Here's the drawing with two shaded views (mm, measured from the low corner). I have some questions. A direction names the side the tool comes from. Give positions to 0.01 mm unless a question says otherwise; leave off trailing zeros. Write each loop counter-clockwise with the first axis right and the second up, starting at its lowest first coordinate (ties: lowest second). Pieces come first, ordered by that corner, then holes.
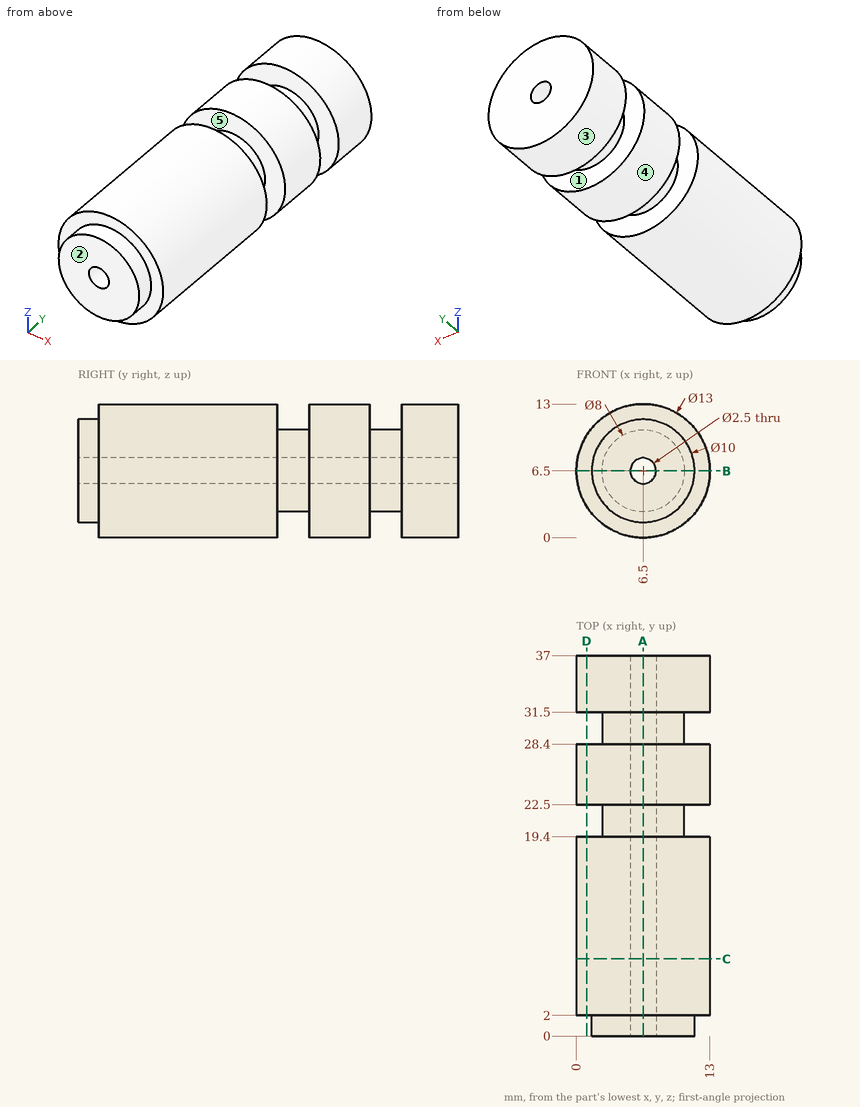
1) For pin 1 Ø1 at (y, z) = (30.5, 10) entering from -X; pin 2 Ø1.5 at (x, y) = (8.5, 26.5) entering from -Z; pin 3 Ø5 at (y, z) = (28, 1.5) entering from -X, each with a flat end and sliding along its axis, tell me the tip position at first contact or that it passes through.
Values follow:
pin 1: stops at x = 3.85
pin 2: stops at z = 0.12
pin 3: stops at x = 0.5
2) Suppose I cut it at C-C on y = 7.5. Write out the boundary of the cut face in (x, z).
Values follow:
outline: circle Ø13 at (6.5, 6.5); hole circle Ø2.5 at (6.5, 6.5)
3) Please list where these lines run through material, in increasing order: L1, parallel to Y at x = 11, z = 3.5; L2, parallel to Y at x = 9.5, z = 3.5; L3, parallel to X at y = 18.5, z = 6.5.
Values follow:
L1: y = 2 to 19.4, 22.5 to 28.4, 31.5 to 37
L2: y = 0 to 19.4, 22.5 to 28.4, 31.5 to 37
L3: x = 0 to 5.25, 7.75 to 13
4) For the marked faces 4 and 5, which set-ups out of +Z, -Z, +X, -X, +Y, -Y let a thin tool reach every point of the face, with its end or its side?
Values follow:
face 4: +Y, -Y
face 5: none
5) Suppose I cut it at D-D on x = 1. Write out the boundary of the cut face in (y, z), plus the area to 3 significant figures.
Values follow:
outline: (2, 3.04) - (19.4, 3.04) - (19.4, 9.96) - (2, 9.96) - close; (22.5, 3.04) - (28.4, 3.04) - (28.4, 9.96) - (22.5, 9.96) - close; (31.5, 3.04) - (37, 3.04) - (37, 9.96) - (31.5, 9.96) - close
area: 200 mm2
6) Suppose I cut it at A-A on x = 6.5. Write out the boundary of the cut face in (y, z).
Values follow:
outline: (0, 1.5) - (2, 1.5) - (2, 0) - (19.4, 0) - (19.4, 2.5) - (22.5, 2.5) - (22.5, 0) - (28.4, 0) - (28.4, 2.5) - (31.5, 2.5) - (31.5, 0) - (37, 0) - (37, 5.25) - (0, 5.25) - close; (0, 7.75) - (37, 7.75) - (37, 13) - (31.5, 13) - (31.5, 10.5) - (28.4, 10.5) - (28.4, 13) - (22.5, 13) - (22.5, 10.5) - (19.4, 10.5) - (19.4, 13) - (2, 13) - (2, 11.5) - (0, 11.5) - close
7) Suppose I cut it at B-B on z = 6.5. Write out the boundary of the cut face in (x, y).
Values follow:
outline: (0, 2) - (1.5, 2) - (1.5, 0) - (5.25, 0) - (5.25, 37) - (0, 37) - (0, 31.5) - (2.5, 31.5) - (2.5, 28.4) - (0, 28.4) - (0, 22.5) - (2.5, 22.5) - (2.5, 19.4) - (0, 19.4) - close; (7.75, 0) - (11.5, 0) - (11.5, 2) - (13, 2) - (13, 19.4) - (10.5, 19.4) - (10.5, 22.5) - (13, 22.5) - (13, 28.4) - (10.5, 28.4) - (10.5, 31.5) - (13, 31.5) - (13, 37) - (7.75, 37) - close
8) If we mould it in two halves opening along Y, with no side actions, what happens to the marked faces 1, 2 and 3? For each: +Y half, -Y half, draft (parallel to the pull), parting line (faces both ways), or undercut.
Values follow:
face 1: undercut
face 2: -Y half
face 3: draft
